Check sheet for the drawn part. Datum: minimum x, y, z corner. Units: mm. Coordinates: 2 decimals unless noted, no trailing zeros. Loops run counter-clockwise (first coordinate to the right, second up) from the corner with the lowest first, then second, coordinate; pieces in that order, holes last. Notation, with made-up numbers: (74, 45) -> (98, 45) arc R20 cw to (98, 60) -> close; hole circle Ø4 at (21.5, -28). An arc over 180 degrees is marked (long way). Use CSV: the item, a comma, the result in double quotes. Start each with the question number.
1. Sectioned sample at A-A, the plane y = 1.45. Count the separate pieces of the cut face and the enclosed holes in it, and give its area (3 significant figures).
2. Gauge pin test, flat end, axial feed: pin 1 (1.9 mm diameter, centred on x = 214.34, z = 6.6, fed in from +Y). Record the tip position at first contact, or that the pin passes through.
3. Thickness scan on L1, parallel to Z at x = 243.4, y = 1.35; L2, parallel to X at y = 0.95, z = 6.6; L3, parallel to X at y = 1.05, z = 25. Record the ranges inside material, lowest first.
4. Sectioned sample at B-B, the plane x = 226. Record the cut outline in (y, z), and give its area (3 significant figures).
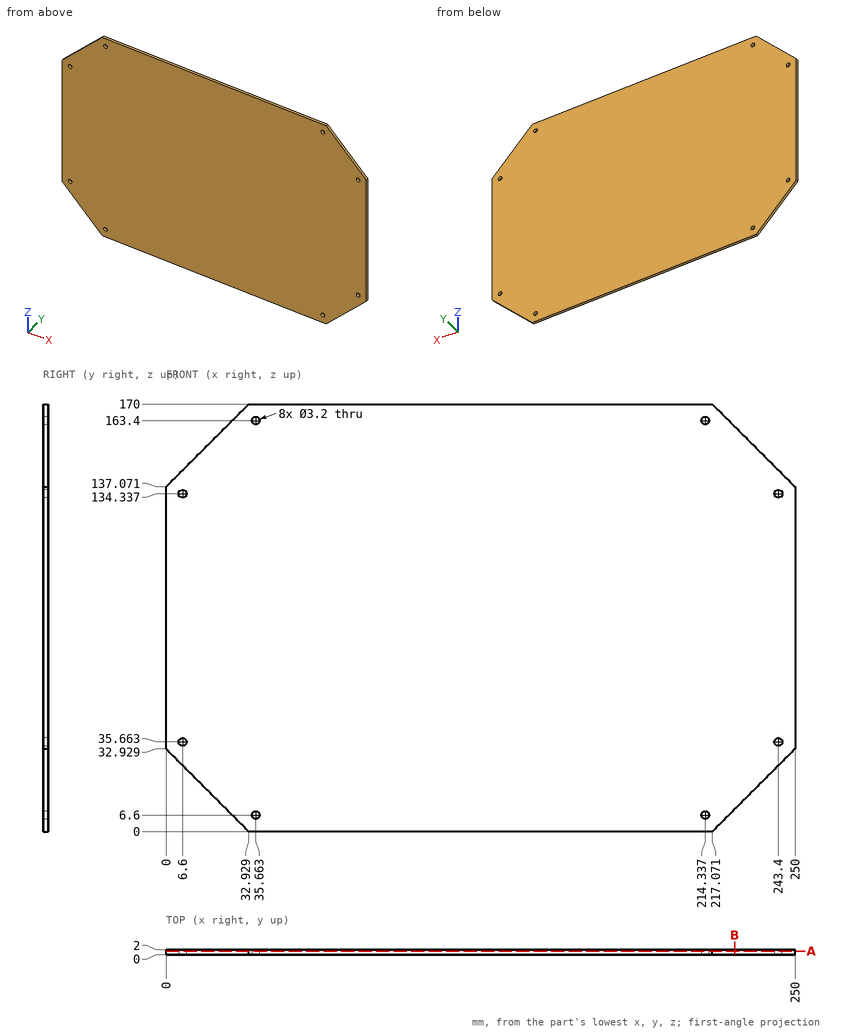
Completed:
1,separate pieces,"1"
1,enclosed holes,"8"
1,area,"40,300 mm²"
2,pin 1,"through"
3,L1,"26.33 to 34.06, 37.26 to 132.74, 135.94 to 143.67"
3,L2,"26.33 to 34.06, 37.26 to 212.74, 215.94 to 223.67"
3,L3,"7.93 to 242.07"
4,outline,"(0, 8.93) -> (2, 8.93) -> (2, 161.07) -> (0, 161.07) -> close"
4,area,"304 mm²"
